Part model, mm, in its own coordinate system. Face numbers are marked on the shaded views. A direction names the side the tool comes from. Give positions to 0.01 mm unless a question says otherwise; leave off trailing zeros. Loops run counter-clockwise (first coordinate to the right, second up) from the corner with the lowest first, then second, coordinate; pieces in that order, holes last. Notation, with made-up numbers: M 20.5,-36 L 45.5,-36 A21 ccw 45.5,-9 Z; hole C 27.5,-8 d6. An arc over 180 degrees is marked long. Put each result on its own line as item: value. Start each with the question number.
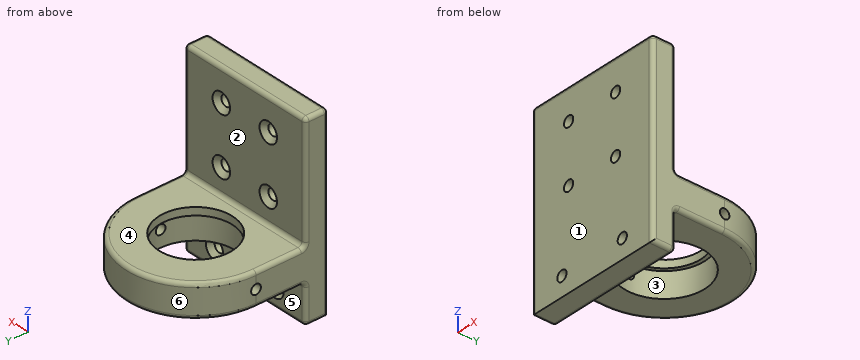
```python
from build123d import *

# Parameters (mm, degrees)
SKETCH1_R                                            = 21
BOSS_EXTRUDE1_DEPTH                                  = 17
BOSS_EXTRUDE2_DEPTH                                  = 60
BOSS_EXTRUDE2_DEPTH_BACK                             = 37
SKETCH2_W                                            = 72
SKETCH2_H                                            = 12
FILLET1_R                                            = 2
BOSS_EXTRUDE4_START                                  = -4
SKETCH4_R                                            = 21
SKETCH4_R_2                                          = 19
BOSS_EXTRUDE4_DEPTH                                  = 4
SKETCH7_R                                            = 2.5
CUT_EXTRUDE3_DEPTH                                   = 112.889454374
CSK_FOR_M5_COUNTERSUNK_RAISED_HEAD_SCREW_D           = 5.5
CSK_FOR_M5_COUNTERSUNK_RAISED_HEAD_SCREW_CSINK_D     = 10.4
CSK_FOR_M5_COUNTERSUNK_RAISED_HEAD_SCREW_CSINK_ANGLE = 90


with BuildPart() as part:
    # Sketch1 → Boss-Extrude1 (new body)
    with BuildSketch(Plane.XY):
        with BuildLine():
            Line((-36, 0), (-36, -37.5))
            Line((-36, -37.5), (36, -37.5))
            Line((36, -37.5), (36, 0))
            ThreePointArc((36, 0), (0, 36), (-36, 0))
        make_face()
        Circle(SKETCH1_R, mode=Mode.SUBTRACT)
    extrude(amount=BOSS_EXTRUDE1_DEPTH)

    # Sketch2 → Boss-Extrude2 (add, two sides: drawn at the far end of the back side and taken through both)
    with BuildSketch(Plane.XY.offset(17).offset(-BOSS_EXTRUDE2_DEPTH_BACK)):
        with Locations((0, -31.5)):
            Rectangle(SKETCH2_W, SKETCH2_H)
    extrude(amount=BOSS_EXTRUDE2_DEPTH + BOSS_EXTRUDE2_DEPTH_BACK)

    # Fillet1
    fillet1_edges = [part.edges().sort_by_distance(p)[0] for p in [
        (36, -12.75, 0),
        (36, -12.75, 17),
        (36, -31.5, -20),
        (36, -25.5, -10),
        (-36, -31.5, -20),
        (0, -25.5, 0),
        (0, -25.5, -20),
        (-36, -25.5, -10),
        (36, -25.5, 47),
        (0, -25.5, 17),
        (-36, -25.5, 47),
        (36, -31.5, 77),
        (0, -25.5, 77),
        (-36, -31.5, 77),
        (0, -37.5, 77),
        (0, 36, 17),
        (-36, -12.75, 0),
        (0, 36, 0),
        (36, -37.5, 28.5),
        (-36, -37.5, 28.5),
        (-36, -12.75, 17),
    ]]
    fillet(fillet1_edges, radius=FILLET1_R)

    # Sketch4 → Boss-Extrude4 (add)
    with BuildSketch(Plane.XY.offset(17).offset(BOSS_EXTRUDE4_START)):
        Circle(SKETCH4_R)
        Circle(SKETCH4_R_2, mode=Mode.SUBTRACT)
    extrude(amount=BOSS_EXTRUDE4_DEPTH)

    # Sketch7 → Cut-Extrude3 (cut, through all)
    with BuildSketch(Plane(origin=(36, 0, 0), x_dir=(0, 0, -1), z_dir=(1, 0, 0))):
        with Locations((-8.5, 0)):
            Circle(SKETCH7_R)
    extrude(amount=-CUT_EXTRUDE3_DEPTH, mode=Mode.SUBTRACT)

    # CSK for M5 Countersunk Raised Head Screw1 (through all)
    with Locations(Plane(origin=(-14, -25.5, 60.144417791), x_dir=(1, 0, 0), z_dir=(0, 1, 0))):
        with Locations((0, 0), (28, 0), (-4, 70.144417791), (32, 70.144417791), (0, 30), (28, 30)):
            CounterSinkHole(CSK_FOR_M5_COUNTERSUNK_RAISED_HEAD_SCREW_D / 2, CSK_FOR_M5_COUNTERSUNK_RAISED_HEAD_SCREW_CSINK_D / 2, counter_sink_angle=CSK_FOR_M5_COUNTERSUNK_RAISED_HEAD_SCREW_CSINK_ANGLE)


solid = part.part
```
1) Which spindle directions (+Z, -Z, +X, -X, +Y, -Y) get a long thin tool onto all of the face, cutting with end or side? Do the marked faces 5 and 6. Say none if no direction does.
2) Band-saw the part on C-C on z = 8.5. Give the cut face in (x, y).
3) Mould opens along Y. For the marked faces 1, 2, 3 and 4 say: +Y half, -Y half, draft (parallel to the pull), parting line (faces both ways), or undercut.
4) Wall check: L1, parallel to Z at x = 14, y = -31.75; L2, parallel to Y at x = 6, z = 25.5; L3, parallel to Y at x = 29.5, z = 8.5. Give the ranges that are in metal, low to high.
5) Band-saw the part on D-D on x = -14. State how many separate pieces and enclosed holes the cut face has, then the cut area to 3 significant figures.
6) Pin check, flat tips, straight feed: pin 1 Ø2 at (x, z) = (-9.5, 35.5) entering from +Y; pin 2 Ø17 at (x, y) = (-14.5, 12.5) entering from -Z; pin 3 Ø3 at (x, y) = (17.5, -25.5) entering from -Z; pin 4 Ø3 at (y, z) = (0, 8.5) entering from +X. Stop position of each tip, or through.
7) Band-saw the part on A-A on z = -10. Give the cut face in (x, y).
8) Band-saw the part on B-B on y = -16. Give the cut face in (x, z), then the cut area to 3 significant figures.
Evaluation:
1. face 5: -Z, +X, -X, +Y
1. face 6: +Z, -Z, +Y
2. outline: M -36,-35.5 A2 ccw -34,-37.5 L 34,-37.5 A2 ccw 36,-35.5 L 36,-2.5 L 20.85,-2.5 A21 cw -20.85,-2.5 L -36,-2.5 Z; M -35.91,2.5 L -20.85,2.5 A21 cw 20.85,2.5 L 35.91,2.5 A36 ccw Z
3. face 1: -Y half
3. face 2: +Y half
3. face 3: undercut
3. face 4: draft
4. L1: -20 to 27.39, 32.89 to 57.39, 62.89 to 77
4. L2: -37.5 to -25.5
4. L3: -37.5 to -2.5, 2.5 to 20.63
5. separate pieces: 4
5. enclosed holes: 0
5. area: 1,500 mm2
6. pin 1: y = -25.5
6. pin 2: z = 0
6. pin 3: z = -19.94
6. pin 4: through
7. outline: M -36,-35.5 A2 ccw -34,-37.5 L -20.75,-37.5 L -20.75,-27.95 L -23.2,-25.5 L -34,-25.5 A2 ccw -36,-27.5 Z; M -15.25,-37.5 L 15.25,-37.5 L 15.25,-27.95 L 12.8,-25.5 L -12.8,-25.5 L -15.25,-27.95 Z; M 20.75,-37.5 L 34,-37.5 A2 ccw 36,-35.5 L 36,-27.5 A2 ccw 34,-25.5 L 23.2,-25.5 L 20.75,-27.95 Z
8. outline: M -36,2 A2 ccw -34,0 L -13.6,0 L -13.6,13 L -10.25,13 L -10.25,17 L -34,17 A2 ccw -36,15 Z; M 10.25,13 L 13.6,13 L 13.6,0 L 34,0 A2 ccw 36,2 L 36,15 A2 ccw 34,17 L 10.25,17 Z
8. area: 785 mm2
